from build123d import *

# Parameters (mm, degrees)
BOSS_EXTRUDE2_DEPTH = 100
CUT_EXTRUDE1_REACH  = 125.859
CUT_EXTRUDE2_REACH  = 115.248


with BuildPart() as part:
    # Sketch1 → Boss-Extrude2 (new body)
    with BuildSketch(Plane(origin=(0, 0, 0), x_dir=(0, 0, -1), z_dir=(1, 0, 0))):
        with BuildLine():
            Line((-19, 70), (-11, 70))
            Line((-11, 70), (-11, 39))
            ThreePointArc((-11, 39), (-9.828427125, 36.171572875), (-7, 35))
            Line((-7, 35), (0, 35))
            Line((0, 35), (0, 0))
            Line((0, 0), (-8, 0))
            Line((-8, 0), (-8, 27))
            Line((-8, 27), (-40, 27))
            Line((-40, 27), (-40, 35))
            Line((-40, 35), (-23, 35))
            ThreePointArc((-23, 35), (-20.171572875, 36.171572875), (-19, 39))
            Line((-19, 39), (-19, 70))
        make_face()
    extrude(amount=BOSS_EXTRUDE2_DEPTH)

    # Sketch2 → Cut-Extrude1 (cut, up to next)
    with BuildSketch(Plane.XY.offset(19), mode=Mode.PRIVATE) as cut_extrude1_sk1:
        with BuildLine():
            Line((14, 56), (14, 70))
            Line((14, 70), (26, 70))
            Line((26, 70), (26, 56))
            ThreePointArc((26, 56), (20, 50), (14, 56))
        make_face()
    cut_extrude1_tool1 = extrude(cut_extrude1_sk1.sketch, amount=-CUT_EXTRUDE1_REACH, mode=Mode.PRIVATE) & part.part
    # Sketch2 → Cut-Extrude1 (cut, up to next)
    with BuildSketch(Plane.XY.offset(19), mode=Mode.PRIVATE) as cut_extrude1_sk2:
        with BuildLine():
            Line((34, 56), (34, 70))
            Line((34, 70), (46, 70))
            Line((46, 70), (46, 56))
            ThreePointArc((46, 56), (40, 50), (34, 56))
        make_face()
    cut_extrude1_tool2 = extrude(cut_extrude1_sk2.sketch, amount=-CUT_EXTRUDE1_REACH, mode=Mode.PRIVATE) & part.part
    # Sketch2 → Cut-Extrude1 (cut, up to next)
    with BuildSketch(Plane.XY.offset(19), mode=Mode.PRIVATE) as cut_extrude1_sk3:
        with BuildLine():
            Line((54, 56), (54, 70))
            Line((54, 70), (66, 70))
            Line((66, 70), (66, 56))
            ThreePointArc((66, 56), (60, 50), (54, 56))
        make_face()
    cut_extrude1_tool3 = extrude(cut_extrude1_sk3.sketch, amount=-CUT_EXTRUDE1_REACH, mode=Mode.PRIVATE) & part.part
    # Sketch2 → Cut-Extrude1 (cut, up to next)
    with BuildSketch(Plane.XY.offset(19), mode=Mode.PRIVATE) as cut_extrude1_sk4:
        with BuildLine():
            Line((74, 56), (74, 70))
            Line((74, 70), (86, 70))
            Line((86, 70), (86, 56))
            ThreePointArc((86, 56), (80, 50), (74, 56))
        make_face()
    cut_extrude1_tool4 = extrude(cut_extrude1_sk4.sketch, amount=-CUT_EXTRUDE1_REACH, mode=Mode.PRIVATE) & part.part
    add(cut_extrude1_tool1.solids().sort_by_distance((20, 60.595886, 19))[0], mode=Mode.SUBTRACT)
    add(cut_extrude1_tool2.solids().sort_by_distance((40, 60.595886, 19))[0], mode=Mode.SUBTRACT)
    add(cut_extrude1_tool3.solids().sort_by_distance((60, 60.595886, 19))[0], mode=Mode.SUBTRACT)
    add(cut_extrude1_tool4.solids().sort_by_distance((80, 60.595886, 19))[0], mode=Mode.SUBTRACT)

    # Sketch3 → Cut-Extrude2 (cut, up to next)
    with BuildSketch(Plane(origin=(0, 35, 0), x_dir=(1, 0, 0), z_dir=(0, 1, 0)), mode=Mode.PRIVATE) as cut_extrude2_sk1:
        with BuildLine():
            Line((20, -40), (80, -40))
            ThreePointArc((80, -40), (77.071067812, -32.928932188), (70, -30))
            Line((70, -30), (30, -30))
            ThreePointArc((30, -30), (22.928932188, -32.928932188), (20, -40))
        make_face()
    cut_extrude2_tool1 = extrude(cut_extrude2_sk1.sketch, amount=-CUT_EXTRUDE2_REACH, mode=Mode.PRIVATE) & part.part
    add(cut_extrude2_tool1.solids().sort_by_distance((50, 35, 35.213132))[0], mode=Mode.SUBTRACT)


solid = part.part
The model under review builds one solid part; all positions refer to its coordinate system, in mm. A direction names the side the tool comes from. Round coordinates to 2 decimals unless told otherwise and drop trailing zeros. Order: outer loops, then holes, each group sorted by start corner. A loop starts at its lowest first (then second) coordinate and runs counter-clockwise, first axis right, second up. Notation, with made-up numbers: (-27, -6) -> (-21, -6) arc R31 ccw to (-21, 33) -> close; hole circle Ø1 at (-18.5, 32). An arc over 180 degrees is marked (long way). Return JSON: item names as keys, results as strings.
1. Take a section at A-A (z = 15). Write out the cut boundary in (x, y), then the cut area to 3 significant figures.
Answer block:
{"outline": "(0, 27) -> (100, 27) -> (100, 70) -> (86, 70) -> (86, 56) arc R6 cw to (74, 56) -> (74, 70) -> (66, 70) -> (66, 56) arc R6 cw to (54, 56) -> (54, 70) -> (46, 70) -> (46, 56) arc R6 cw to (34, 56) -> (34, 70) -> (26, 70) -> (26, 56) arc R6 cw to (14, 56) -> (14, 70) -> (0, 70) -> close", "area": "3,400 mm²"}
2. Take a section at D-D (z = 35). Write out the cut boundary in (x, y), then the cut area to 3 significant figures.
Answer block:
{"outline": "(0, 27) -> (21.34, 27) -> (21.34, 35) -> (0, 35) -> close; (78.66, 27) -> (100, 27) -> (100, 35) -> (78.66, 35) -> close", "area": "341 mm²"}
3. For faces 4 (the face through (49, 35, 4)), 5 (the face through (54, 63, 15)), 6 (the face through (49.3, 35, 29.7)), 7 (the face through (77.15, 31.06, 33.01)), list the 3-axis set-ups (+Z, -Z, +X, -X, +Y, -Y) from which the entire face can be reached by the end or side of a thin tool; tool diameter is ignored.
Answer block:
{"face 4": "-Z, +X, -X, +Y", "face 5": "+Z, -Z, +Y", "face 6": "+Z, +X, -X, +Y", "face 7": "+Z, +Y, -Y"}
4. Take a section at C-C (y = 30.5). Write out the cut boundary in (x, z), then the cut area to 3 significant figures.
Answer block:
{"outline": "(0, 0) -> (100, 0) -> (100, 40) -> (80, 40) arc R10 cw to (70, 30) -> (30, 30) arc R10 cw to (20, 40) -> (0, 40) -> close", "area": "3,440 mm²"}
5. The part is to be moulded in two halves that separate along Z. For faces 1 (the face through (66, 63, 15)), 2 (the face through (49.3, 36.203, 9.859)), 3 (the face through (49.3, 36.141, 20.203)), say which applies: +Z half, -Z half, draft (parallel to the pull), parting line (faces both ways), or undercut.
Answer block:
{"face 1": "draft", "face 2": "-Z half", "face 3": "+Z half"}
6. Insertion check: P1, Ø3, axis at x = 62, y = 8.5, coming from the +Z side; P2, Ø9.5, axis at x = 27, z = 22.5, coming from the -Y side; P3, Ø2.5, axis at x = 50.5, y = 31.5, coming from the +Z side; P4, Ø2, axis at y = 43.5, z = 9, coming from the -X side. Each pin has a flat end and moves straight along its axis. Give the tip position at first contact, or say it passes through.
Answer block:
{"P1": "stops at z = 8", "P2": "stops at y = 27", "P3": "stops at z = 30", "P4": "passes through"}
7. For L1, parallel to X at y = 65.5, z = 15; L2, parallel to X at y = 52.5, z = 14.5; L3, parallel to Z at x = 50, y = 13.5, list the stretches that pass through material, from the lowest coordinate up. Write a range as [from, to].
Answer block:
{"L1": "x = [0, 14], [26, 34], [46, 54], [66, 74], [86, 100]", "L2": "x = [0, 15.13], [24.87, 35.13], [44.87, 55.13], [64.87, 75.13], [84.87, 100]", "L3": "z = [0, 8]"}
8. Take a section at B-B (x = 40). Write out the cut boundary in (y, z), then the cut area to 3 significant figures.
Answer block:
{"outline": "(0, 0) -> (35, 0) -> (35, 7) arc R4 cw to (39, 11) -> (50, 11) -> (50, 19) -> (39, 19) arc R4 cw to (35, 23) -> (35, 30) -> (27, 30) -> (27, 8) -> (0, 8) -> close", "area": "583 mm²"}
